Geometry check sheet. Reference: the model listing, model coordinates, mm. Coordinates: 2 decimals unless noted, no trailing zeros. Order: outer loops, then holes, each group sorted by start corner. A loop starts at its lowest first (then second) coordinate and runs counter-clockwise, first axis right, second up.
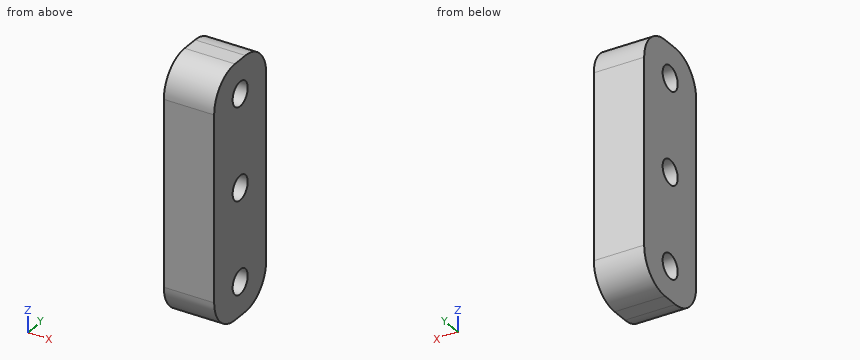
```python
from build123d import *

# Parameters (mm, degrees)
SKETCH1_W           = 30
SKETCH1_H           = 10
BOSS_EXTRUDE1_DEPTH = 6
SKETCH2_R           = 1.45
CUT_EXTRUDE1_DEPTH  = 33.186953879
FILLET1_R           = 4


with BuildPart() as part:
    # Sketch1 → Boss-Extrude1 (new body)
    with BuildSketch(Plane(origin=(0, 0, 0), x_dir=(0, 0, -1), z_dir=(1, 0, 0))):
        with Locations((15, -5)):
            Rectangle(SKETCH1_W, SKETCH1_H)
    extrude(amount=BOSS_EXTRUDE1_DEPTH)

    # Sketch2 → Cut-Extrude1 (cut, through all)
    with BuildSketch(Plane(origin=(6, 0, 0), x_dir=(0, 0, -1), z_dir=(1, 0, 0))):
        with Locations((4, -5)):
            Circle(SKETCH2_R)
        with Locations((15, -5)):
            Circle(SKETCH2_R)
        with Locations((26, -5)):
            Circle(SKETCH2_R)
    extrude(amount=-CUT_EXTRUDE1_DEPTH, mode=Mode.SUBTRACT)

    # Fillet1
    fillet1_edges = [part.edges().sort_by_distance(p)[0] for p in [
        (3, 0, 0),
        (3, 0, -30),
        (3, -10, -30),
        (3, -10, 0),
    ]]
    fillet(fillet1_edges, radius=FILLET1_R)


solid = part.part
```
Item 1: Sectioned sample at C-C (y = -5). Record the cut outline in (x, z).
Item 2: Sectioned sample at D-D (y = -7.75). Record the cut outline in (x, z).
Item 3: Depth check by flat-ended pin: P1, Ø2.5, axis at y = -5, z = -15, coming from the +X side; P2, Ø1.5, axis at x = 3.5, y = -7.5, coming from the -Z side. Enter the tip coordinate at first touch or a pass-through.
Item 4: Sectioned sample at B-B (x = 3.7). Record the cut outline in (y, z), and give its area (3 significant figures).
Item 5: Thickness scan on line 1 along Y through (x, z) = (2.85, -15); line 2 along Z through (x, y) = (2.15, -4.5); line 3 along Z through (x, y) = (5.5, -7.75). Record the ranges inside material, lowest first.
Item 6: Sectioned sample at A-A (z = -15). Record the cut outline in (x, y).
Geometry check:
1. outline: (0, -30) - (6, -30) - (6, -27.45) - (0, -27.45) - close; (0, -24.55) - (6, -24.55) - (6, -16.45) - (0, -16.45) - close; (0, -13.55) - (6, -13.55) - (6, -5.45) - (0, -5.45) - close; (0, -2.55) - (6, -2.55) - (6, 0) - (0, 0) - close
2. outline: (0, -29.6) - (6, -29.6) - (6, -0.4) - (0, -0.4) - close
3. P1: passes through
3. P2: stops at z = -29.93
4. outline: (-10, -26) arc R4 ccw to (-6, -30) - (-4, -30) arc R4 ccw to (0, -26) - (0, -4) arc R4 ccw to (-4, 0) - (-6, 0) arc R4 ccw to (-10, -4) - close; hole circle Ø2.9 at (-5, -26); hole circle Ø2.9 at (-5, -15); hole circle Ø2.9 at (-5, -4)
4. area: 266 mm2
5. line 1: y = -10 to -6.45, -3.55 to 0
5. line 2: z = -30 to -27.36, -24.64 to -16.36, -13.64 to -5.36, -2.64 to 0
5. line 3: z = -29.6 to -0.4
6. outline: (0, -10) - (6, -10) - (6, -6.45) - (0, -6.45) - close; (0, -3.55) - (6, -3.55) - (6, 0) - (0, 0) - close
